Source: CAD feature listing. Evaluate the final solid. Frame: model axes, mm. Give positions to 0.01 mm unless a question says otherwise; leave off trailing zeros. Order: outer loops, then holes, each group sorted by start corner. A loop starts at its lowest first (then second) coordinate and runs counter-clockwise, first axis right, second up. Notation, with made-up numbers: (57.25, 1) - (83.25, 1) arc R13 cw to (83.25, 17) - close; hole circle Ø6 at (74, 87). An arc over 180 degrees is marked (long way). Use CSV: the item, a comma, the result in double quotes.
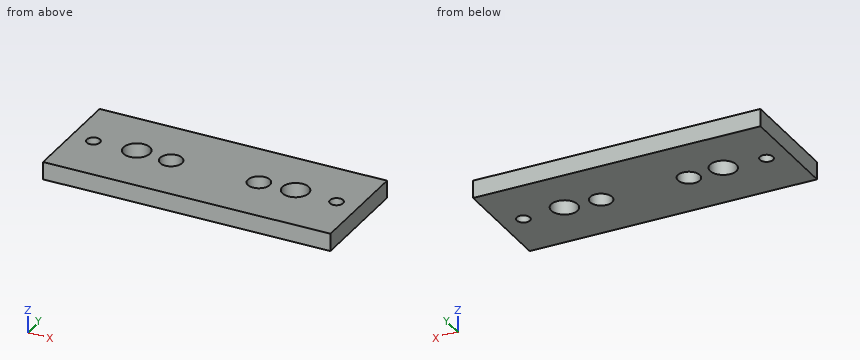
```python
from build123d import *

# Parameters (mm, degrees)
SKETCH1_W             = 65.5
SKETCH1_H             = 25
BOSS_EXTRUDE1_DEPTH   = 4
F_5_0MM_DOWEL_HOLE1_D = 5
SKETCH4_R             = 3
CUT_EXTRUDE1_DEPTH    = 71.222859526
F_3_0MM_DOWEL_HOLE1_D = 3


with BuildPart() as part:
    # Sketch1 → Boss-Extrude1 (new body)
    with BuildSketch(Plane.XY):
        with Locations((32.75, 12.5)):
            Rectangle(SKETCH1_W, SKETCH1_H)
    extrude(amount=BOSS_EXTRUDE1_DEPTH)

    # Ø5.0mm Dowel Hole1 (through all)
    with Locations(Plane.XY.offset(4)):
        with Locations((22.75, 12.5), (42.75, 12.5)):
            Hole(F_5_0MM_DOWEL_HOLE1_D / 2)

    # Sketch4 → Cut-Extrude1 (cut, through all)
    with BuildSketch(Plane.XY.offset(4)):
        with Locations((14.65, 13)):
            Circle(SKETCH4_R)
        with Locations((50.85, 13)):
            Circle(SKETCH4_R)
    extrude(amount=-CUT_EXTRUDE1_DEPTH, mode=Mode.SUBTRACT)

    # Ø3.0mm Dowel Hole1 (through all)
    with Locations(Plane.XY.offset(4)):
        with Locations((5.05, 12.5), (60.45, 12.5)):
            Hole(F_3_0MM_DOWEL_HOLE1_D / 2)


solid = part.part
```
Item 1: Section A-A on x = 42.75. Return the cut outline in (y, z), then the cut area to 3 significant figures.
Filled in:
outline,"(0, 0) - (10, 0) - (10, 4) - (0, 4) - close; (15, 0) - (25, 0) - (25, 4) - (15, 4) - close"
area,"80.0 mm2"
Item 2: Material intervals for line 1 (Y direction, x = 14.65, z = 1.85); line 2 (Y direction, x = 14, z = 1.65), sorted ascending. Write a range as from..to.
Filled in:
line 1,"y = 0..10, 16..25"
line 2,"y = 0..10.07, 15.93..25"
Item 3: Section C-C on x = 5.05. Return the cut outline in (y, z), then the cut area to 3 significant figures.
Filled in:
outline,"(0, 0) - (11, 0) - (11, 4) - (0, 4) - close; (14, 0) - (25, 0) - (25, 4) - (14, 4) - close"
area,"88.0 mm2"
Item 4: First-contact query: pin 1 (3.5 mm diameter, centred on x = 60.45, y = 12.5, fed in from -Z). Flat tip, straight axial feed; report the tip coordinate or a pass-through.
Filled in:
pin 1,"stops at z = 0"
Item 5: Section B-B on z = 1. Return the cut outline in (x, y), then the cut area to 3 significant figures.
Filled in:
outline,"(0, 0) - (65.5, 0) - (65.5, 25) - (0, 25) - close; hole circle Ø3 at (5.05, 12.5); hole circle Ø6 at (14.65, 13); hole circle Ø5 at (22.75, 12.5); hole circle Ø5 at (42.75, 12.5); hole circle Ø6 at (50.85, 13); hole circle Ø3 at (60.45, 12.5)"
area,"1,530 mm2"
